Design review of the part built by this model. Coordinates are the model's own, in mm. A direction names the side the tool comes from. Coordinates: 2 decimals unless noted, no trailing zeros. Loops run counter-clockwise (first coordinate to the right, second up) from the corner with the lowest first, then second, coordinate; pieces in that order, holes last. Notation, with made-up numbers: (71, -1.5) - (103, -1.5) arc R13 cw to (103, 12.5) - close; hole circle Ø3 at (28, 5.25). An arc over 180 degrees is marked (long way). Answer in a Markdown table with one row per item. Add a question column.
(1) The part is to be moulded in two halves that separate along Y. For faces 5 (the face through (0, 150, -6)), 6 (the face through (16.2, 127, -2)), 7 (the face through (4, 148.79, 3)), say which applies: released by +Y, released by -Y, zero draft, split by the parting line, or undercut.
(2) For faces 1 (the face through (0, -148.79, 0)), 2 (the face through (0, 2, -11.29)), 3 (the face through (0, -2, -12.5)), 4 (the face through (-2.192, 149.403, -4.214)), list the 3-axis set-ups (+Z, -Z, +X, -X, +Y, -Y) from which the entire face can be reached by the end or side of a thin tool; tool diameter is ignored.
(3) We need section A-A, the plane x = 0. Write out the cut boundary in (y, z), plus the area to 3 significant figures.
(4) To check wall thickness, follow L1, parallel to Y at x = 11, z = -9.75; L2, parallel to Z at x = 15.55, y = -112.5 (3 decimals); L3, parallel to Z at x = 0, y = 149.45. State the ranges of each line that lie inside material, in increasing order. Write a range as [from, to].
(5) We need section C-C, the plane y = 101. Write out the cut boundary in (x, z).
(6) We need section B-B, the plane x = -12. Write out the cut boundary in (y, z).
(7) Clearance check with flat-ended pins moving along their axes: pin 1 (1.6 mm diameter, centred on y = -149, z = -4, fed in from +X); pin 2 (10 mm diameter, centred on x = -4.5, y = 65, fed in from +Z); pin 3 (1 mm diameter, centred on x = 15.5, y = -123.5, fed in from +Z); pin 4 (2.5 mm diameter, centred on y = -112.5, z = -3.5, fed in from -X). State where each tip first meets the part, or that it passes through.
from build123d import *

# Parameters (mm, degrees)
F1_DEPTH = 15
F3_W     = 41
F3_H     = 20
F4_DEPTH = 1.2
F2_R     = 4.75
F5_DEPTH = 1.21
F6_R     = 1.385
F7_DEPTH = 1.2


with BuildPart() as f1:
    # F0 (on Right) → F1 (new body, symmetric)
    with BuildSketch(Plane.YZ):
        Polygon((-148.79, 12.5), (-150, 12.5), (-150, -12.5), (150, -12.5), (150, 12.5), (148.79, 12.5), (148.79, -11.29), (0, -11.29), (-148.79, -11.29), align=None)
    extrude(amount=F1_DEPTH, both=True)

    # F3 (on face) → F4 (join)
    with BuildSketch(Plane.YZ.offset(15)):
        with Locations((-127.5, -2.5)):
            Rectangle(F3_W, F3_H)
        with Locations((127.5, -2.5)):
            Rectangle(F3_W, F3_H)
    extrude(amount=F4_DEPTH)

    # F2 (on face) → F5 (cut, through all)
    with BuildSketch(Plane(origin=(0, 150, 0), x_dir=(-1, 0, 0), z_dir=(0, 1, 0))):
        Circle(F2_R)
    extrude(amount=-F5_DEPTH, mode=Mode.SUBTRACT)

    # F6 (on face) → F7 (cut, through all)
    with BuildSketch(Plane.YZ.offset(16.2)):
        with Locations((-112.5, -3.5)):
            Circle(F6_R)
        with Locations((112.5, -3.5)):
            Circle(F6_R)
    extrude(amount=-F7_DEPTH, mode=Mode.SUBTRACT)


solid = f1.part
Responses:
| question | item | result |
|---|---|---|
| 1 | face 5 | released by +Y |
| 1 | face 6 | zero draft |
| 1 | face 7 | undercut |
| 2 | face 1 | +Z, +X, -X |
| 2 | face 2 | +Z, -X |
| 2 | face 3 | -Z, +X, -X, +Y, -Y |
| 2 | face 4 | +Y |
| 3 | outline | (-150, -12.5) - (150, -12.5) - (150, -4.75) - (148.79, -4.75) - (148.79, -11.29) - (-148.79, -11.29) - (-148.79, 12.5) - (-150, 12.5) - close; (148.79, 4.75) - (150, 4.75) - (150, 12.5) - (148.79, 12.5) - close |
| 3 | area | 409 mm2 |
| 4 | L1 | y = [-150, -148.79], [148.79, 150] |
| 4 | L2 | z = [-12.5, -4.885], [-2.115, 7.5] |
| 4 | L3 | z = [-12.5, -4.75], [4.75, 12.5] |
| 5 | outline | (-15, -12.5) - (15, -12.5) - (15, -11.29) - (-15, -11.29) - close |
| 6 | outline | (-150, -12.5) - (150, -12.5) - (150, 12.5) - (148.79, 12.5) - (148.79, -11.29) - (-148.79, -11.29) - (-148.79, 12.5) - (-150, 12.5) - close |
| 7 | pin 1 | stops at x = 15 |
| 7 | pin 2 | stops at z = -11.29 |
| 7 | pin 3 | stops at z = 7.5 |
| 7 | pin 4 | passes through |
